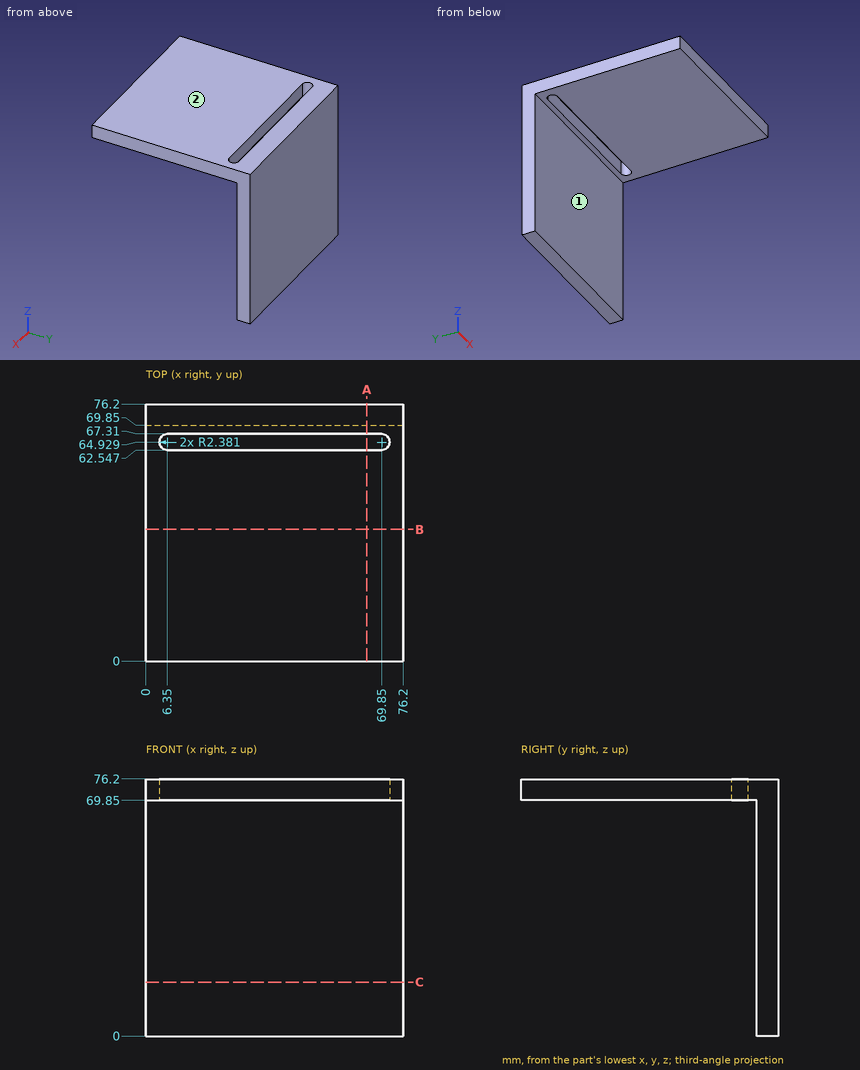
The figure shows three views and two pictorial views of one solid part (mm, origin at its lowest corner). Answer the questions. A direction names the side the tool comes from. Coordinates: 2 decimals unless noted, no trailing zeros. Loops run counter-clockwise (first coordinate to the right, second up) from the corner with the lowest first, then second, coordinate; pieces in that order, holes last. Notation, with made-up numbers: (-11.5, 63) - (-2.5, 63) arc R5 cw to (-2.5, 68) - close; hole circle Ø6 at (81, 25.25). An arc over 180 degrees is marked (long way). Use a Markdown table: item, result. Add a question column.
1) Given pin 1 (6 mm diameter, centred on x = 46, z = 16.5, fed in from -Y); pin 2 (12 mm diameter, centred on x = 19.5, y = 58, fed in from -Z), each flat-ended and moving along its own axis, determine where each tip first touches the part or whether it passes through.
2) The part is cut by section A-A, the plane x = 65.5. Give the vertices of the cut face in (y, z), and give its area (3 significant figures).
3) Find the intervals of material crossed by line 1 (Y direction, x = 44, z = 71.5); line 2 (Z direction, x = 65, y = 25), in increasing order.
4) The part is cut by section B-B, the plane y = 39. Give the vertices of the cut face in (x, z).
5) For the marked faces 1 and 2, determine the directions among +Z, -Z, +X, -X, +Y, -Y from which every point of the face is accessible in a straight line to the end or side of a thin tool.
Here are the results:
| question | item | result |
|---|---|---|
| 1 | pin 1 | stops at y = 69.85 |
| 1 | pin 2 | stops at z = 69.85 |
| 2 | outline | (0, 69.85) - (62.55, 69.85) - (62.55, 76.2) - (0, 76.2) - close; (67.31, 69.85) - (69.85, 69.85) - (69.85, 0) - (76.2, 0) - (76.2, 76.2) - (67.31, 76.2) - close |
| 2 | area | 897 mm^2 |
| 3 | line 1 | y = 0 to 62.55, 67.31 to 76.2 |
| 3 | line 2 | z = 69.85 to 76.2 |
| 4 | outline | (0, 69.85) - (76.2, 69.85) - (76.2, 76.2) - (0, 76.2) - close |
| 5 | face 1 | -Z, +X, -X, -Y |
| 5 | face 2 | +Z, +X, -X, +Y, -Y |
